Build history of the part. All positions in model axes, mm. Face numbers are marked on the shaded views. Round coordinates to 2 decimals unless told otherwise and drop trailing zeros. Loops run counter-clockwise (first coordinate to the right, second up) from the corner with the lowest first, then second, coordinate; pieces in that order, holes last. Notation, with made-up numbers: M 61,-28.75 L 118,-28.75 A9 cw 118,-14.75 Z; hole C -13.75,-14.75 d6. An arc over 180 degrees is marked long. Write each question's results on one line, items separated by ' | '. Start each with the question number.
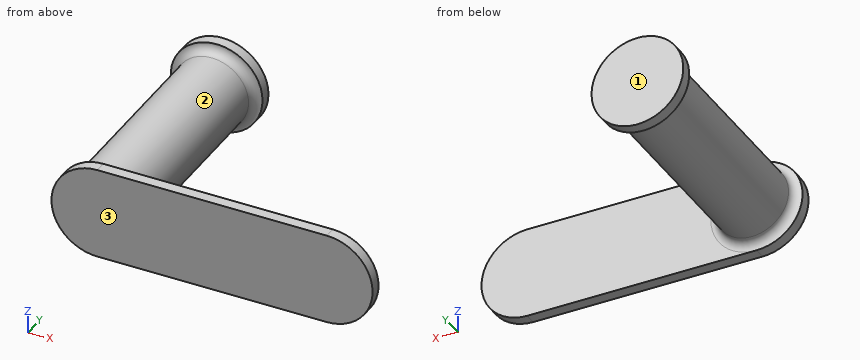
```python
from build123d import *

# Parameters (mm, degrees)
EXTRUDE_1_DEPTH = 5


with BuildPart() as part:
    # 草图1 → 旋转1 (revolve)
    with BuildSketch(Plane.XY):
        with BuildLine():
            Line((0, 60.184685033), (0, -39.815314967))
            Line((0, -39.815314967), (20, -39.815314967))
            ThreePointArc((20, -39.815314967), (17.171572875, -38.643742092), (16, -35.815314967))
            Line((16, -35.815314967), (16, 51.184685033))
            ThreePointArc((16, 51.184685033), (17.171572875, 54.013112157), (20, 55.184685033))
            Line((20, 55.184685033), (20, 60.184685033))
            Line((20, 60.184685033), (0, 60.184685033))
        make_face()
    revolve(axis=Axis((0, 60.184685033, 0), (0, -1, 0)))

    # 草图2 → 凸台-拉伸1 (add)
    with BuildSketch(Plane.XZ.offset(39.815314967)):
        with BuildLine():
            Line((0, -20), (100, -20))
            ThreePointArc((100, -20), (120, 0), (100, 20))
            Line((100, 20), (0, 20))
            ThreePointArc((0, 20), (-20, 0), (0, -20))
        make_face()
    extrude(amount=EXTRUDE_1_DEPTH)


solid = part.part
```
Item 1: Saw through at B-B, the plane y = -25. Give the cut face in (x, z), then the cut area to 3 significant figures.
Item 2: Drop flat-ended pins along their axis: pin 1 (5 mm diameter, centred on x = -5.5, y = 8, fed in from -Z); pin 2 (4 mm diameter, centred on x = 77.5, z = 12.5, fed in from +Y); pin 3 (5 mm diameter, centred on y = 9, z = 2, fed in from -X). Give the stop position or say it passes through.
Item 3: Mould opens along Y. For the marked faces 1, 2 and 3 say: released by +Y, released by -Y, zero draft, split by the parting line, or undercut.
Item 4: Saw through at A-A, the plane z = 0. Give the cut face in (x, y).
Item 5: Drill centre lines: line 1 along Y through (x, z) = (36, -13); line 2 along Z through (x, y) = (-0.5, 43); line 3 along X through (y, z) = (4.5, -13.5). Where is each one in solid material? Low to high. Write a range as [from, to].
Item 6: Saw through at C-C, the plane x = 81. Give the cut face in (y, z), then the cut area to 3 significant figures.
Working result:
1) outline: C 0,0 d32 | area: 804 mm²
2) pin 1: stops at z = -15.72 | pin 2: stops at y = -39.82 | pin 3: stops at x = -16
3) face 1: released by +Y | face 2: undercut | face 3: released by -Y
4) outline: M -20,-44.82 L 120,-44.82 L 120,-39.82 L 20,-39.82 A4 cw 16,-35.82 L 16,51.18 A4 cw 20,55.18 L 20,60.18 L -20,60.18 L -20,55.18 A4 cw -16,51.18 L -16,-35.82 A4 cw -20,-39.82 Z
5) line 1: y = [-44.82, -39.82] | line 2: z = [-15.99, 15.99] | line 3: x = [-8.59, 8.59]
6) outline: M -44.82,-20 L -39.82,-20 L -39.82,20 L -44.82,20 Z | area: 200 mm²
